Check sheet for the drawn part. Datum: minimum x, y, z corner. Units: mm. A direction names the side the tool comes from. Round coordinates to 2 decimals unless told otherwise and drop trailing zeros. Loops run counter-clockwise (first coordinate to the right, second up) from the corner with the lowest first, then second, coordinate; pieces in that order, holes last. Notation, with made-up numbers: (88.5, 87) - (131.5, 87) arc R20 cw to (131.5, 109) - close; hole circle Ø3 at (-10.5, -26.75). An arc over 180 degrees is marked (long way). Use CSV: the item, a comma, the result in double quotes.
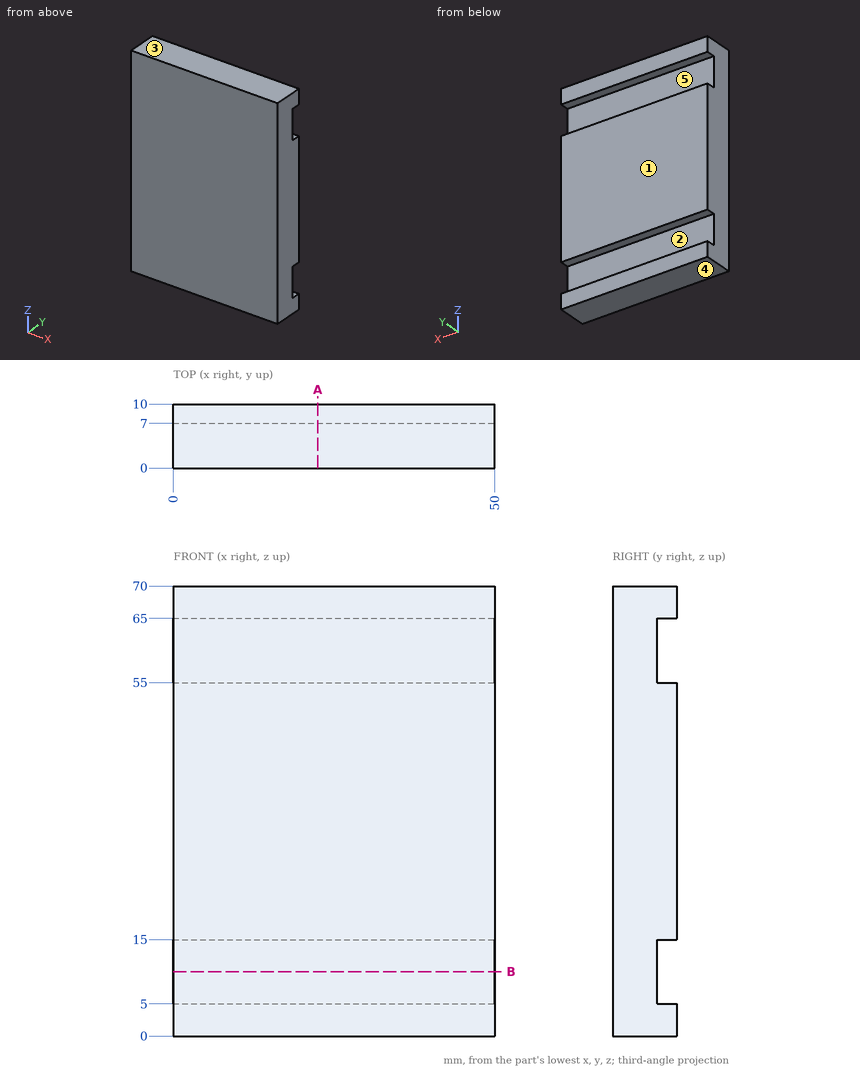
1) Cross-section at B-B, the plane z = 10. Record the cut outline in (x, y).
Returned:
outline,"(0, 0) - (50, 0) - (50, 7) - (0, 7) - close"
2) Gauge pin test, flat end, axial feed: pin 1 Ø12 at (x, z) = (28.5, 14.5) entering from -Y. Record the tip position at first contact, or that the pin passes through.
Returned:
pin 1,"stops at y = 0"
3) Mould release check, pull along Z, two halves, no side actions. Record for the marked faces 1, 2 and 3: +Z half, -Z half, draft (parallel to the pull), parting line (faces both ways), or undercut.
Returned:
face 1,"draft"
face 2,"undercut"
face 3,"+Z half"
4) Access from +Z, -Z, +X, -X, +Y, -Y to the whole of each face (thin tool, end or side, straight path). Record for the marked faces 4 and 5.
Returned:
face 4,"-Z, +X, -X, +Y, -Y"
face 5,"+X, -X, +Y"
5) Cross-section at A-A, the plane x = 22.5. Record the cut outline in (y, z), then the cut area to 3 significant figures.
Returned:
outline,"(0, 0) - (10, 0) - (10, 5) - (7, 5) - (7, 15) - (10, 15) - (10, 55) - (7, 55) - (7, 65) - (10, 65) - (10, 70) - (0, 70) - close"
area,"640 mm²"
6) Thickness scan on probe 1 along Z at (x, y) = (25.5, 7.75); probe 2 along Y at (x, z) = (23.5, 62). Record the ranges inside material, lowest first. Write a range as [from, to].
Returned:
probe 1,"z = [0, 5], [15, 55], [65, 70]"
probe 2,"y = [0, 7]"
